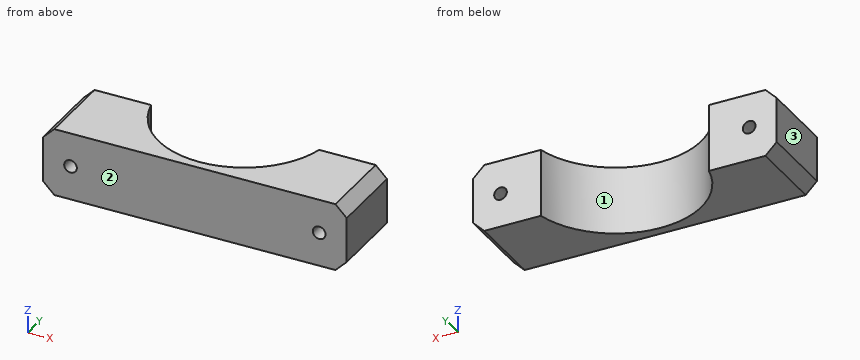
from build123d import *

# Parameters (mm, degrees)
BOSS_EXTRUDE1_DEPTH = 15
CHAMFER1_SIZE       = 2.5
SKETCH2_R           = 1.4
CUT_EXTRUDE1_DEPTH  = 41.512038564


with BuildPart() as part:
    # Sketch1 → Boss-Extrude1 (new body)
    with BuildSketch(Plane.XY):
        with BuildLine():
            Line((-18.574175621, -4), (-33.574175621, -4))
            Line((-33.574175621, -4), (-33.574175621, -21))
            Line((-33.574175621, -21), (33.574175621, -21))
            Line((33.574175621, -21), (33.574175621, -4))
            Line((33.574175621, -4), (18.574175621, -4))
            ThreePointArc((18.574175621, -4), (0, -19), (-18.574175621, -4))
        make_face()
    extrude(amount=BOSS_EXTRUDE1_DEPTH)

    # Chamfer1
    chamfer1_edges = [part.edges().sort_by_distance(p)[0] for p in [
        (-33.574175621, -12.5, 15),
        (33.574175621, -12.5, 15),
        (-33.574175621, -12.5, 0),
        (33.574175621, -12.5, 0),
    ]]
    chamfer(chamfer1_edges, length=CHAMFER1_SIZE)

    # Sketch2 → Cut-Extrude1 (cut, through all)
    with BuildSketch(Plane(origin=(0, -4, 0), x_dir=(1, 0, 0), z_dir=(0, 1, 0))):
        with Locations(Location((27.488644481, -7.5, 0), (0, 0, 180))):
            Circle(SKETCH2_R)
        with Locations((-27.488644481, -7.5)):
            Circle(SKETCH2_R)
    extrude(amount=-CUT_EXTRUDE1_DEPTH, mode=Mode.SUBTRACT)


solid = part.part
Source: CAD feature listing. Evaluate the final solid. Frame: model axes, mm. Face numbers are marked on the shaded views. Give positions to 0.01 mm unless a question says otherwise; leave off trailing zeros. Write each loop counter-clockwise with the first axis right and the second up, starting at its lowest first coordinate (ties: lowest second). Pieces come first, ordered by that corner, then holes. Notation, with made-up numbers: (-26, 67.25) - (-17, 67.25) arc R21 cw to (-17, 95.25) - close; hole circle Ø5 at (-4, 20.5). An arc over 180 degrees is marked (long way). Write item = value, one per line. Start each with the question number.
Q1. Material intervals for probe 1 along Y at (x, z) = (0, 11.75); probe 2 along X at (y, z) = (-19.75, 8.75); probe 3 along X at (y, z) = (-6, 11), sorted ascending.
Q2. Draft query along X for the marked faces 1, 2 and 3. Return one class per face: +X half, -X half, draft (parallel to the pull), parting line (faces both ways), or undercut.
Q3. Pin query (flat end, axial travel): pin 1 Ø5 at (x, z) = (-13, 1.5) entering from +Y; pin 2 Ø2.5 at (x, z) = (-27.49, 7.5) entering from -Y. Return the tip coordinate at first contact, or that it passes through.
Q4. Cut plane B-B, the plane y = -6.75. Return loops of the section in (x, z), then the cut area to 3 significant figures.
Q5. Cut plane A-A, the plane z = 7.5. Return loops of the section in (x, y), then the cut area to 3 significant figures.
Q6. Cut plane D-D, the plane z = 4. Return loops of the section in (x, y).
Q7. Cut plane C-C, the plane y = -11. Return loops of the section in (x, z), then the cut area to 3 significant figures.
Computed values:
q1.probe_1 = -21 to -19
q1.probe_2 = -33.57 to -28.12, -26.86 to 26.86, 28.12 to 33.57
q1.probe_3 = -33.57 to -18.03, 18.03 to 33.57
q2.face_1 = undercut
q2.face_2 = draft
q2.face_3 = -X half
q3.pin_1 = -10.99
q3.pin_2 = through
q4.outline = (-33.57, 2.5) - (-31.07, 0) - (-17.76, 0) - (-17.76, 15) - (-31.07, 15) - (-33.57, 12.5) - close; (17.76, 0) - (31.07, 0) - (33.57, 2.5) - (33.57, 12.5) - (31.07, 15) - (17.76, 15) - close; hole circle Ø2.8 at (-27.49, 7.5); hole circle Ø2.8 at (27.49, 7.5)
q4.area = 450 mm²
q5.outline = (-33.57, -21) - (-28.89, -21) - (-28.89, -4) - (-33.57, -4) - close; (-26.09, -21) - (26.09, -21) - (26.09, -4) - (18.57, -4) arc R19 cw to (-18.57, -4) - (-26.09, -4) - close; (28.89, -21) - (33.57, -21) - (33.57, -4) - (28.89, -4) - close
q5.area = 630 mm²
q6.outline = (-33.57, -21) - (33.57, -21) - (33.57, -4) - (18.57, -4) arc R19 cw to (-18.57, -4) - (-33.57, -4) - close
q7.outline = (-33.57, 2.5) - (-31.07, 0) - (-15.49, 0) - (-15.49, 15) - (-31.07, 15) - (-33.57, 12.5) - close; (15.49, 0) - (31.07, 0) - (33.57, 2.5) - (33.57, 12.5) - (31.07, 15) - (15.49, 15) - close; hole circle Ø2.8 at (-27.49, 7.5); hole circle Ø2.8 at (27.49, 7.5)
q7.area = 518 mm²
